Can you work these out from the model? Positions are in its coordinate system, mm. A direction names the side the tool comes from. Give positions to 0.01 mm unless a question says otherwise; leave off trailing zeros. Loops run counter-clockwise (first coordinate to the right, second up) from the corner with the lowest first, then second, coordinate; pieces in that order, holes last. Notation, with made-up numbers: M -16.75,77 L 9.25,77 A10 ccw 9.25,86 Z; hole C -7,3 d5. An arc over 180 degrees is marked long. Answer as a JSON object with one key per item and string values.
```python
from build123d import *

# Parameters (mm, degrees)
F1_R     = 3.175
F2_DEPTH = 1.5875
F1_W     = 12.7
F1_H     = 1.5875
F3_DEPTH = 26.9875
F4_R     = 3.175
F5_DEPTH = 1.5875
F6_R     = 1.58102


with BuildPart() as f2:
    # F1 (on offset) → F2 (new body)
    with BuildSketch(Plane.XZ.offset(1.5875)):
        Polygon((6.35, 0), (0, 0), (-6.35, 0), (-6.35, -23.8125), (6.35, -23.8125), align=None)
        with Locations((0, -6.35)):
            Circle(F1_R, mode=Mode.SUBTRACT)
    extrude(amount=-F2_DEPTH)

    # F1 (on offset) → F3 (join)
    with BuildSketch(Plane.XZ.offset(1.5875)):
        with Locations((0, -24.60625)):
            Rectangle(F1_W, F1_H)
    extrude(amount=-F3_DEPTH)

    # F4 (on face) → F5 (cut)
    with BuildSketch(Plane.XY.offset(-23.8125)):
        with Locations((0, 19.05)):
            Circle(F4_R)
    extrude(amount=-F5_DEPTH, mode=Mode.SUBTRACT)

    # F6
    f6_edges = [f2.edges().sort_by_distance(p)[0] for p in [
        (0, -1.5875, -25.4),
    ]]
    fillet(f6_edges, radius=F6_R)


solid = f2.part
```
1) Will these pins go through, and if not, where does the flat tip stop? pin 1 Ø5.5 at (x, z) = (0, -6.35) entering from +Y; pin 2 Ø3 at (x, z) = (-2.5, -14) entering from +Y; pin 3 Ø2 at (x, z) = (-0.5, -4) entering from -Y.
Answer list:
{"pin 1": "through", "pin 2": "y = 0", "pin 3": "y = -1.59"}
2) Suppose I cut it at C-C, the plane x = 0. Write out the boundary of the cut face in (y, z) (1 decimal), and give its area (3 significant figures).
Answer list:
{"outline": "M -1.6,-23.8 A1.6 ccw 0,-25.4 L 15.9,-25.4 L 15.9,-23.8 L 0,-23.8 L 0,-9.5 L -1.6,-9.5 Z; M -1.6,-3.2 L 0,-3.2 L 0,0 L -1.6,0 Z; M 22.2,-25.4 L 25.4,-25.4 L 25.4,-23.8 L 22.2,-23.8 Z", "area": "59.9 mm^2"}
3) Please list where these lines run through material, in increasing order: line 1 along Y through (x, z) = (-2.75, -15.75); line 2 along Z through (x, y) = (5.25, 9.5); line 3 along Y through (x, z) = (0, -24.3) (3 decimals). Write a range as from..to.
Answer list:
{"line 1": "-1.59..0", "line 2": "-25.4..-23.81", "line 3": "-1.513..15.875, 22.225..25.4"}
4) For faces 4 (the cylindrical face through (-0.69, 15.95, -24.6)), 5 (the flat face through (0, 0, -12)), which set-ups out of +Z, -Z, +X, -X, +Y, -Y let a thin tool reach every point of the face, with its end or its side?
Answer list:
{"face 4": "+Z, -Z", "face 5": "+Z, +X, -X, +Y"}
5) If we mould it in two halves opening along Z, with no side actions, what happens to faces 1 (the flat face through (0, 13, -23.812)), 2 (the cylindrical face through (-0.69, -0.8, -9.45)), 3 (the flat face through (6.35, 6, -24))? For each: +Z half, -Z half, draft (parallel to the pull), parting line (faces both ways), or undercut.
Answer list:
{"face 1": "+Z half", "face 2": "undercut", "face 3": "draft"}
6) Suppose I cut it at D-D, the plane x = 3.5. Write out the boundary of the cut face in (y, z), and give its area (3 significant figures).
Answer list:
{"outline": "M -1.59,-23.82 A1.58 ccw -0.01,-25.4 L 25.4,-25.4 L 25.4,-23.81 L 0,-23.81 L 0,0 L -1.59,0 Z", "area": "80.1 mm^2"}
